Build history of the part. All positions in model axes, mm. Face numbers are marked on the shaded views. A direction names the side the tool comes from. Round coordinates to 2 decimals unless told otherwise and drop trailing zeros. Write each loop counter-clockwise with the first axis right and the second up, starting at its lowest first coordinate (ties: lowest second). Pieces come first, ordered by that corner, then holes.
1) Wall check: probe 1 along Y at (x, z) = (0, -43) (3 decimals); probe 2 along Y at (x, z) = (-11, -34.5); probe 3 along Y at (x, z) = (7.5, -2). Give the ranges that are in metal, low to high.
2) Flat gauge pins, fed straight in: pin 1 (1 mm diameter, centred on x = 42, z = -41.5, fed in from +Y); pin 2 (2 mm diameter, centred on x = 26, y = 40, fed in from +Z); pin 3 (2 mm diameter, centred on x = -26.5, z = -30.5, fed in from -Y). Where does each tip first touch, or does it go through?
3) Which spindle directions (+Z, -Z, +X, -X, +Y, -Y) get a long thin tool onto all of the face, cutting with end or side? Do the marked faces 1 and 2. Say none if no direction does.
4) Saw through at B-B (y = 0). Write the cut outline in (x, z) (3 decimals).
5) Saw through at C-C (z = -26.5). Write the cut outline in (x, y) (3 decimals).
6) Saw through at D-D (z = -42.5). State how many separate pieces and enclosed holes the cut face has, plus the area to 3 significant figures.
7) Saw through at A-A (x = 0). Write the cut outline in (y, z) (3 decimals).
8) Pull direction Y, two halves, no side cores. Call the marked faces 3, 4 and 5: +Y half, -Y half, draft (parallel to the pull), parting line (faces both ways), or undercut.
Autodesk Inventor part; units mm, degrees
ref_plane "YZ Plane" through (0, 0, 0) normal (1, 0, 0) x (0, 1, 0)
ref_plane "XZ Plane" through (0, 0, 0) normal (0, 1, 0) x (-1, 0, 0)
ref_plane "XY Plane" through (0, 0, 0) normal (0, 0, 1) x (1, 0, 0)
sketch "Sketch1" plane through (0, 0, 0) normal (1, 0, 0) x (0, 1, 0)
  line L0 (0, 0) -> (38.1, 0)
  line L1 (38.1, 0) -> (38.1, -39.624)
  line L2 (38.1, -39.624) -> (68.58, -39.624)
  line L3 (68.58, -39.624) -> (68.58, -46.228)
  line L4 (68.58, -46.228) -> (32.512, -46.228)
  line L5 (32.512, -46.228) -> (32.512, -51.308)
  line L6 (32.512, -51.308) -> (28.448, -51.308)
  line L7 (28.448, -51.308) -> (28.448, -64.516)
  line L8 (28.448, -64.516) -> (0, -64.516)
  line L9 (0, -64.516) -> (0, 0)
  dimension "d0" = 38.1
  dimension "d1" = 39.624
  dimension "d2" = 30.48
  dimension "d3" = 6.604
  dimension "d4" = 36.068
  dimension "d5" = 5.08
  dimension "d6" = 4.064
  dimension "d7" = 13.208
revolve "Revolution1" add sketch "Sketch1" angle 360 about axis through (0, 0, -64.516) along (0, 0, 1)
sketch "Sketch2" plane through (0, 0, -64.516) normal (0, 0, -1) x (-1, 0, 0)
  circle A0 centre (0, 0) radius 25.4
  dimension "d9" = 50.8
extrude "Extrusion1" cut sketch "Sketch2" against normal up to surface (18.288 mm away)
sketch "Sketch3" plane through (0, 0, -46.228) normal (0, 0, -1) x (-1, 0, 0)
  circle A0 centre (0, 0) radius 15.875
  dimension "d12" = 31.75
extrude "Extrusion2" cut sketch "Sketch3" against normal up to surface (46.228 mm away)
fillet "Fillet1" radius 1.905 2 edges at (0, -28.448, -51.308) (0, -32.512, -46.228)
chamfer "Chamfer1" distance 0.762 angle 45 5 edges at (0, -68.58, -46.228) (0, -68.58, -39.624) (0, -38.1, 0) (0, -32.512, -51.308) (0, -28.448, -64.516)
fillet "Fillet2" radius 6.35 1 edges at (0, -38.1, -39.624)
sketch "Sketch4" plane through (0, 0, -39.624) normal (0, 0, 1) x (1, 0, 0)
  line L0 (1.6378, 0) -> (0, 0)
  line L1 (0, 0) -> (0, 80.9396)
  circle A0 centre (0, 56.388) radius 5.7404
  circle A1 centre (0, 0) radius 68.58
  line L2 (0, 68.58) -> (-43.6157, 68.58)
  circle A2 centre (53.6282, 17.4249) radius 5.7404
  circle A3 centre (33.144, -45.6189) radius 5.7404
  circle A4 centre (-33.144, -45.6189) radius 5.7404
  circle A5 centre (-53.6282, 17.4249) radius 5.7404
  line L3 (0, 0) -> (47.9546, 47.9546)
  circle A6 centre (0, 0) radius 67.818
  line L4 (0, 0) -> (67.818, 0) construction
  circle A7 centre (0, 0) radius 44.45
  arc A8 (53.6282, 17.4249) -> (0, 56.388) centre (0, 0) ccw
  circle A9 centre (39.8723, 39.8723) radius 2.54
  dimension "d20" = 11.4808
  dimension "d21" = 12.192
  dimension "d24" = 360
  dimension "d26" = 45
  dimension "d27" = 5.08
extrude "Extrusion3" cut sketch "Sketch4" against normal up to surface (6.604 mm away) contours A2 | A0 L1 | L1 A8 A0 | A9 A8 L3 | L3 A8 A9 | L1 A0 A8 | A8 A9 L3 | L3 A9 A8 | A3 | A4 | A5
thread "Thread1"
thread "Thread2"
thread "Thread3"
thread "Thread4"
thread "Thread5"
thread "Thread6"
sketch "Sketch5" plane through (0, 0, -46.228) normal (0, 0, -1) x (-1, 0, 0)
  circle A0 centre (0, 0) radius 44.45
  point P0 (0, 0)
extrude "Extrusion4" cut sketch "Sketch5" along normal up to surface (18.288 mm away)
sketch "Sketch6" plane through (0, 0, -39.624) normal (0, 0, 1) x (1, 0, 0)
  circle A0 centre (0, 56.388) radius 5.7404
  circle A1 centre (0, 0) radius 56.388
  circle A2 centre (39.8723, 39.8723) radius 2.54
  circle A3 centre (39.8723, 39.8723) radius 4.1275
  circle A4 centre (-25.5996, 50.2421) radius 4.1275
  circle A5 centre (-55.6938, -8.821) radius 4.1275
  circle A6 centre (-8.821, -55.6938) radius 4.1275
  circle A7 centre (50.2421, -25.5996) radius 4.1275
  point P0 (0, 0)
  dimension "d44" = 8.255
  dimension "d47" = 360
extrude "Extrusion5" cut sketch "Sketch6" against normal blind 25.4 contours A4 A1 | A1 A4 | A3 A1 A2 | A1 A2 A3 | A5 A1 | A1 A5 | A7 A1 | A1 A7 | A6 A1 | A1 A6
thread "Thread7"
thread "Thread8"
thread "Thread9"
thread "Thread10"
thread "Thread11"
equation "\"d28\" = d27"
properties part number "DTR-1"
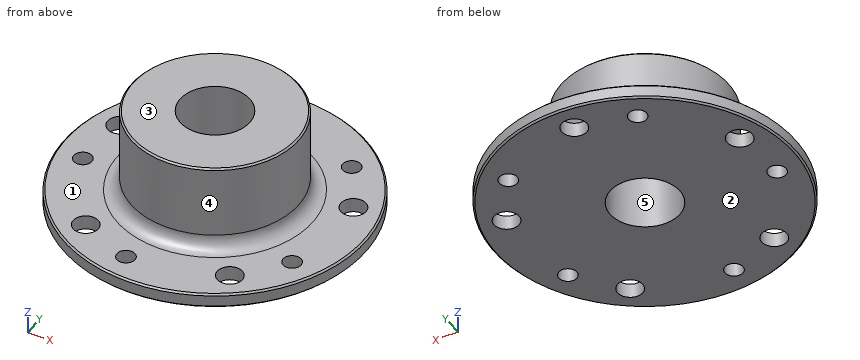
Evaluation:
1. probe 1: y = -68.58 to -15.875, 15.875 to 50.648, 62.128 to 68.58
1. probe 2: y = -36.6 to -11.45, 11.45 to 36.6
1. probe 3: y = -37.35 to -13.99, 13.99 to 37.35
2. pin 1: stops at y = 54.6
2. pin 2: stops at z = -39.62
2. pin 3: stops at y = -28.31
3. face 1: +Z
3. face 2: -Z, +X, -X, +Y, -Y
4. outline: (-68.58, -45.466) - (-67.818, -46.228) - (-15.875, -46.228) - (-15.875, 0) - (-37.338, 0) - (-38.1, -0.762) - (-38.1, -33.274) arc R6.35 cw to (-44.45, -39.624) - (-67.818, -39.624) - (-68.58, -40.386) - close; (15.875, -46.228) - (67.818, -46.228) - (68.58, -45.466) - (68.58, -40.386) - (67.818, -39.624) - (44.45, -39.624) arc R6.35 cw to (38.1, -33.274) - (38.1, -0.762) - (37.338, 0) - (15.875, 0) - close
5. outline: circle Ø76.2 at (0, 0); hole circle Ø31.75 at (0, 0)
6. separate pieces: 1
6. enclosed holes: 11
6. area: 13,200 mm2
7. outline: (-68.58, -45.466) - (-67.818, -46.228) - (-15.875, -46.228) - (-15.875, 0) - (-37.338, 0) - (-38.1, -0.762) - (-38.1, -33.274) arc R6.35 cw to (-44.45, -39.624) - (-67.818, -39.624) - (-68.58, -40.386) - close; (15.875, -46.228) - (50.648, -46.228) - (50.648, -39.624) - (44.45, -39.624) arc R6.35 cw to (38.1, -33.274) - (38.1, -0.762) - (37.338, 0) - (15.875, 0) - close; (62.128, -46.228) - (67.818, -46.228) - (68.58, -45.466) - (68.58, -40.386) - (67.818, -39.624) - (62.128, -39.624) - close
8. face 3: draft
8. face 4: parting line
8. face 5: undercut
